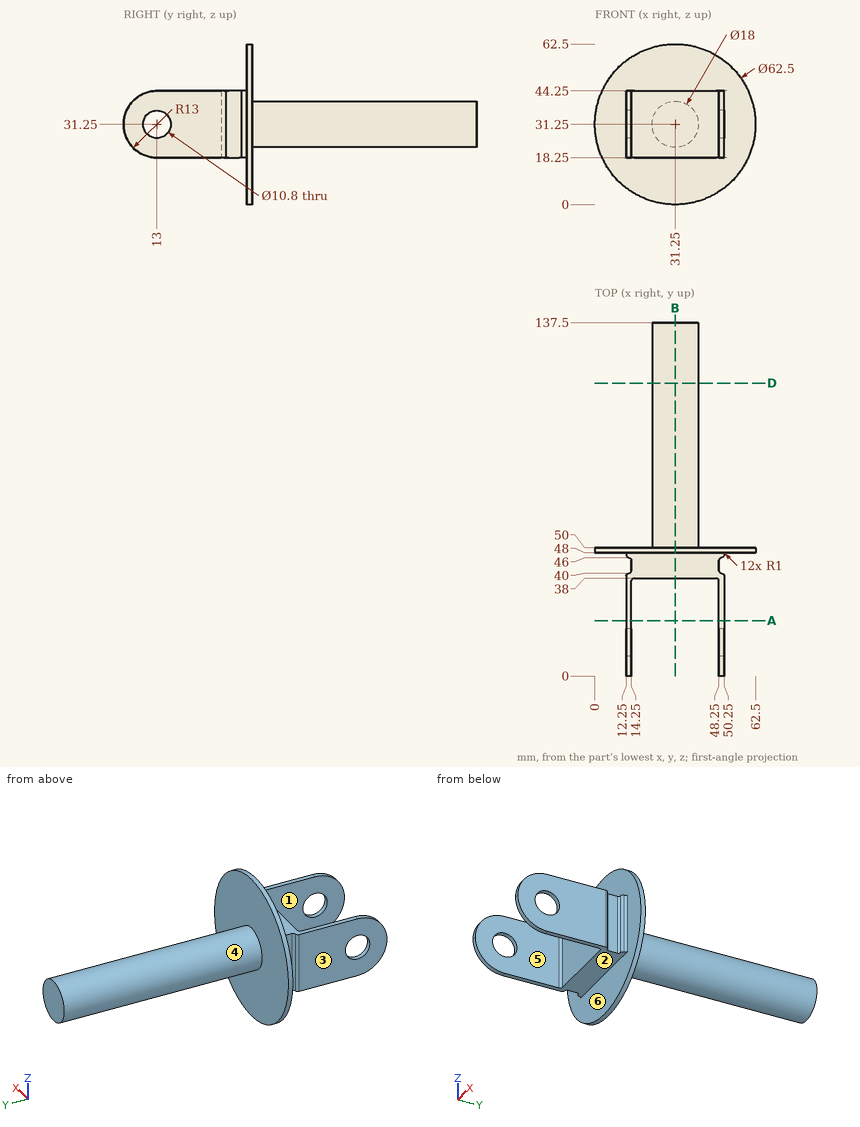
Part print with two shaded views. Sizes in mm from the minimum x, y, z corner. A direction names the side the tool comes from. Coordinates: 2 decimals unless noted, no trailing zeros. Loops run counter-clockwise (first coordinate to the right, second up) from the corner with the lowest first, then second, coordinate; pieces in that order, holes last. Notation, with made-up numbers: (-2.75, 26.25) -> (14.25, 26.25) arc R18 cw to (14.25, 59.25) -> close; hole circle Ø1 at (16, 73.25). An arc over 180 degrees is marked (long way). Answer as a JSON object with one key per item and string values.
Q1. Cut at D-D (y = 114). List the corners of the cut face in (x, z), and give its area (3 significant figures).
Report:
{"outline": "circle Ø18 at (31.25, 31.25)", "area": "254 mm2"}
Q2. 3-axis set-ups, long thin cutter, end or side, ignore diameter. For the marked faces 4, 5 and 6: which of +Z, -Z, +X, -X, +Y, -Y reach the whole face in a straight line?
Report:
{"face 4": "+Y", "face 5": "+Z, -Z, -Y", "face 6": "-Y"}
Q3. Flat gauge pins, fed straight in: P1, Ø21, axis at y = 9.5, z = 36, coming from the +X side; P2, Ø6, axis at y = 53.5, z = 10.5, coming from the -X side; P3, Ø2, axis at y = 42.5, z = 37.5, coming from the +X side; P4, Ø21, axis at y = 26, z = 25, coming from the -X side. Where does each tip first touch, or does it go through?
Report:
{"P1": "stops at x = 50.25", "P2": "passes through", "P3": "stops at x = 48.25", "P4": "stops at x = 12.25"}
Q4. Pull direction X, two halves, no side cores. Call the marked faces 1, 2 and 3: released by +X, released by -X, zero draft, split by the parting line, or undercut.
Report:
{"face 1": "undercut", "face 2": "zero draft", "face 3": "released by -X"}
Q5. Probe probe 1 along Y at (x, z) = (49.2, 31.25); probe 2 along X at (y, z) = (10, 23); probe 3 along Y at (x, z) = (52.5, 33). List the from-to ranges inside material, lowest first.
Report:
{"probe 1": "y = 0 to 7.6, 18.4 to 40, 46 to 50", "probe 2": "x = 12.25 to 14.25, 48.25 to 50.25", "probe 3": "y = 48 to 50"}
Q6. Cut at B-B (x = 31.25). List the corners of the cut face in (y, z), and give its area (3 significant figures).
Report:
{"outline": "(38, 18.25) -> (48, 18.25) -> (48, 0) -> (50, 0) -> (50, 22.25) -> (137.5, 22.25) -> (137.5, 40.25) -> (50, 40.25) -> (50, 62.5) -> (48, 62.5) -> (48, 44.25) -> (38, 44.25) -> close", "area": "1,960 mm2"}
Q7. Cut at A-A (y = 21.5). List the corners of the cut face in (x, z), and give its area (3 significant figures).
Report:
{"outline": "(12.25, 18.25) -> (14.25, 18.25) -> (14.25, 44.25) -> (12.25, 44.25) -> close; (48.25, 18.25) -> (50.25, 18.25) -> (50.25, 44.25) -> (48.25, 44.25) -> close", "area": "104 mm2"}
